Verification items for the finished model (mm, model axes). A direction names the side the tool comes from. Coordinates: 2 decimals unless noted, no trailing zeros. Order: outer loops, then holes, each group sorted by start corner. A loop starts at its lowest first (then second) coordinate and runs counter-clockwise, first axis right, second up. Notation, with made-up numbers: M -16,1 L 38,1 A19 ccw 38,13 Z; hole C 40,-35.5 d2. An arc over 180 degrees is marked long. Return JSON: item names as keys, results as strings.
```python
from build123d import *

# Parameters (mm, degrees)
SKETCH2_R           = 50.75
SKETCH2_R_2         = 35.5
BOSS_EXTRUDE1_DEPTH = 20
SKETCH3_R           = 2.75
CUT_EXTRUDE1_DEPTH  = 251.172565442
SKETCH4_R           = 5
CUT_EXTRUDE2_DEPTH  = 10
BOSS_EXTRUDE2_START = 3
SKETCH5_R           = 20
SKETCH5_R_2         = 30
BOSS_EXTRUDE2_DEPTH = 3
CHAMFER1_SIZE       = 0.7
CHAMFER2_SIZE       = 0.5


with BuildPart() as part:
    # Sketch2 → Boss-Extrude1 (new body)
    with BuildSketch(Plane.XY):
        with BuildLine():
            Line((-10.1, 109), (-10.1, 129.1))
            Line((-10.1, 129.1), (10.1, 129.1))
            Line((10.1, 129.1), (10.1, 109))
            Line((10.1, 109), (60, 109))
            ThreePointArc((60, 109), (85.993749249, 175.900264083), (21.650423731, 144.1))
            Line((21.650423731, 144.1), (-19.589286853, 144.1))
            ThreePointArc((-19.589286853, 144.1), (-100.713392844, 206.860656309), (-70, 109))
            Line((-70, 109), (-10.1, 109))
        make_face()
        with Locations((-70, 162.75)):
            Circle(SKETCH2_R, mode=Mode.SUBTRACT)
        with Locations((60, 147.5)):
            Circle(SKETCH2_R_2, mode=Mode.SUBTRACT)
    extrude(amount=BOSS_EXTRUDE1_DEPTH)

    # Sketch3 → Cut-Extrude1 (cut, through all)
    with BuildSketch(Plane(origin=(0, 0, 0), x_dir=(1, 0, 0), z_dir=(0, 1, 0))):
        with Locations(Location((0, -10, 0), (0, 0, 90))):
            Circle(SKETCH3_R)
    extrude(amount=CUT_EXTRUDE1_DEPTH, mode=Mode.SUBTRACT)

    # Sketch4 → Cut-Extrude2 (cut)
    with BuildSketch(Plane(origin=(0, 144.1, 0), x_dir=(1, 0, 0), z_dir=(0, 1, 0))):
        with Locations(Location((0, -10, 0), (0, 0, 270))):
            Circle(SKETCH4_R)
    extrude(amount=-CUT_EXTRUDE2_DEPTH, mode=Mode.SUBTRACT)

    # Sketch5 → Boss-Extrude2 (add)
    with BuildSketch(Plane(origin=(0, 0, 0), x_dir=(-1, 0, 0), z_dir=(0, 0, -1)).offset(BOSS_EXTRUDE2_START)):
        with BuildLine():
            Line((10.1, 109), (70, 109))
            ThreePointArc((70, 109), (100.713392844, 206.860656309), (19.589286853, 144.1))
            Line((19.589286853, 144.1), (-21.650423731, 144.1))
            ThreePointArc((-21.650423731, 144.1), (-85.993749249, 175.900264083), (-60, 109))
            Line((-60, 109), (-10.1, 109))
            Line((-10.1, 109), (-10.1, 129.1))
            Line((-10.1, 129.1), (10.1, 129.1))
            Line((10.1, 129.1), (10.1, 109))
        make_face()
        with Locations((-60, 147.5)):
            Circle(SKETCH5_R, mode=Mode.SUBTRACT)
        with Locations((70, 162.75)):
            Circle(SKETCH5_R_2, mode=Mode.SUBTRACT)
    extrude(amount=-BOSS_EXTRUDE2_DEPTH)

    # Chamfer1
    chamfer1_edges = [part.edges().sort_by_distance(p)[0] for p in [
        (-10.1, 119.05, -3),
        (-40.05, 109, -3),
        (-100.713392844, 206.860656309, -3),
        (1.030568439, 144.1, -3),
        (85.993749249, 175.900264083, -3),
        (35.05, 109, -3),
        (10.1, 119.05, -3),
        (0, 129.1, -3),
        (80, 147.5, -3),
        (-40, 162.75, -3),
    ]]
    chamfer(chamfer1_edges, length=CHAMFER1_SIZE)

    # Chamfer2
    chamfer2_edges = [part.edges().sort_by_distance(p)[0] for p in [
        (0, 129.1, 20),
        (10.1, 109, 10),
        (-10.1, 109, 8.85),
        (10.1, 119.05, 20),
        (35.05, 109, 20),
        (-120.75, 162.75, 20),
        (85.993749249, 175.900264083, 20),
        (24.5, 147.5, 20),
        (1.030568439, 144.1, 20),
        (-100.713392844, 206.860656309, 20),
        (-40.05, 109, 20),
        (-10.1, 119.05, 20),
    ]]
    chamfer(chamfer2_edges, length=CHAMFER2_SIZE)


solid = part.part
```
Q1. Tool access check on faces 4 (the face through (-11, 140, -3)), 5 (the face through (-92, 141, 0)), 6 (the face through (1.5, 139.17, 14.77)). Record the directions out of +Z, -Z, +X, -X, +Y, -Y that give a thin tool (end or side, any length) a straight path to the whole face; none if there is none.
Values:
{"face 4": "-Z, +X, -X, +Y, -Y", "face 5": "+Z", "face 6": "+Y"}
Q2. Cross-section at A-A, the plane x = 0. Record the boundary of the cut face in (y, z), and give its area (3 significant figures).
Values:
{"outline": "M 129.1,-2.3 L 129.8,-3 L 143.4,-3 L 144.1,-2.3 L 144.1,5 L 134.1,5 L 134.1,7.25 L 129.1,7.25 Z; M 129.1,12.75 L 134.1,12.75 L 134.1,15 L 144.1,15 L 144.1,19.5 L 143.6,20 L 129.6,20 L 129.1,19.5 Z", "area": "217 mm^2"}
Q3. Go/stop test with flat-tipped pins: pin 1 (2.5 mm diameter, centred on x = -4.5, z = -1, fed in from -Y); pin 2 (1.5 mm diameter, centred on y = 144, z = 9, fed in from +X); pin 3 (1.8 mm diameter, centred on y = 117.5, z = -1.5, fed in from -X). Record where each tip stops, or that it passes through.
Values:
{"pin 1": "y = 129.1", "pin 2": "x = 98.4", "pin 3": "x = -100.37"}
Q4. Material ranges on line 1 along X through (y, z) = (170, 15); line 2 along X through (y, z) = (146, 5.25); line 3 along Y through (x, z) = (-70, -0.9), recorded low to high.
Values:
{"line 1": "-123.26 to -120.23, -19.77 to -16.74, 28.76 to 32.54, 87.46 to 91.24", "line 2": "-121.07 to -117.91, -22.09 to -18.93, 21.53 to 24.53, 95.47 to 98.47", "line 3": "109 to 132.75, 192.75 to 216.5"}
Q5. Draft check along Z on faces 1 (the face through (86.49, 174.94, 19.86)), 2 (the face through (-2.2, 134.1, 12.2)), 3 (the face through (-10.1, 119, 8)). Enter one of: pulls with the +Z half, pulls with the -Z half, needs draft (parallel to the pull), parting line crosses it, or undercut.
Values:
{"face 1": "pulls with the +Z half", "face 2": "undercut", "face 3": "needs draft"}
Q6. Cross-section at B-B, the plane y = 150. State how many separate pieces and enclosed holes the cut face has, and give its area (3 significant figures).
Values:
{"separate pieces": "4", "enclosed holes": "0", "area": "503 mm^2"}
